Answer from the drawing. Dimensions are ordinates in mm from the lowest x, y and z of the part. A direction names the side the tool comes from. Give positions to 0.01 mm unless a question says otherwise; leave off trailing zeros. Write each loop counter-clockwise with the first axis right and the second up, starting at its lowest first coordinate (ties: lowest second). Pieces come first, ordered by that corner, then holes. Notation, with made-up numbers: (-18, 75) - (6, 75) arc R19 cw to (6, 109) - close; hole circle Ø1 at (-9.5, 49). An arc over 180 degrees is marked (long way). Write item = value, one per line.
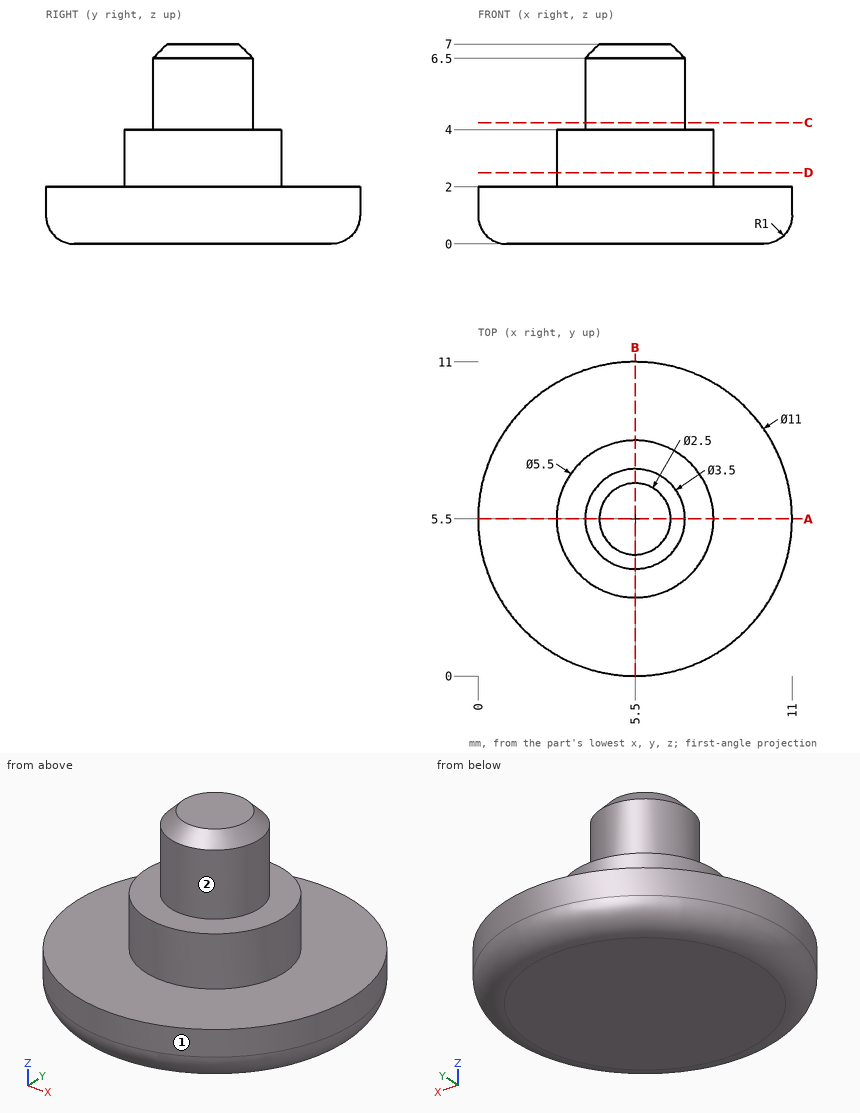
1. A tool of negligible diameter and unlimited length cuts with its end or side. For the marked faces 1 and 2, from which of +Z, -Z, +X, -X, +Y, -Y can it reach the whole face along a straight path? Write none if from no direction.
Solution:
face_1 = +Z, -Z
face_2 = +Z
2. Find section A-A, the plane y = 5.5. Give the vertices of the cut face in (x, z).
Solution:
outline = (0, 1) arc R1 ccw to (1, 0) - (10, 0) arc R1 ccw to (11, 1) - (11, 2) - (8.25, 2) - (8.25, 4) - (7.25, 4) - (7.25, 6.5) - (6.75, 7) - (4.25, 7) - (3.75, 6.5) - (3.75, 4) - (2.75, 4) - (2.75, 2) - (0, 2) - close
3. Find section D-D, the plane z = 2.5. Give the vertices of the cut face in (x, y), then the cut area to 3 significant figures.
Solution:
outline = circle Ø5.5 at (5.5, 5.5)
area = 23.8 mm^2
4. Straight lines are drawn through the part: line 1 (Z direction, x = 4, y = 5.5); line 2 (Z direction, x = 4, y = 8.5); line 3 (Y direction, x = 5.5, z = 6). For each, find the intervals that lie inside material, in ascending order.
Solution:
line_1 = 0 to 6.75
line_2 = 0 to 2
line_3 = 3.75 to 7.25
5. Find section C-C, the plane z = 4.25. Give the vertices of the cut face in (x, y).
Solution:
outline = circle Ø3.5 at (5.5, 5.5)
6. Given pin 1 (1 mm diameter, centred on y = 4.5, z = 5.5, fed in from +X); pin 2 (1.5 mm diameter, centred on y = 2.5, z = 5, fed in from +X); pin 3 (2 mm diameter, centred on x = 8.5, z = 4.5, fed in from -Y), each flat-ended and moving along its own axis, determine where each tip first touches the part or whether it passes through.
Solution:
pin_1 = 7.18
pin_2 = through
pin_3 = 3.77
